Check sheet for the modelled part. Datum: model origin and axes. Units: mm. Round coordinates to 2 decimals unless told otherwise and drop trailing zeros. Loops run counter-clockwise (first coordinate to the right, second up) from the corner with the lowest first, then second, coordinate; pieces in that order, holes last. Notation, with made-up numbers: (77.25, -16) - (83.25, -16) arc R17 ccw to (83.25, -9) - close; hole circle Ø6 at (70.5, 10). An arc over 180 degrees is marked (long way). Return JSON: item names as keys, results as strings.
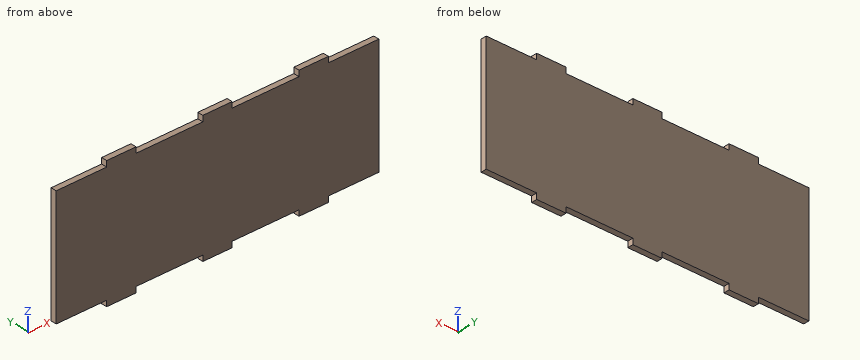
Autodesk Fusion 360 part; units mm, degrees
sketch "Skizze1" plane through (0, 0, 0) normal (0, 1, 0) x (1, 0, 0)
  line L0 (0, 0) -> (101, 0)
  line L1 (101, 0) -> (101, 40.6)
  line L2 (101, 40.6) -> (0, 40.6)
  line L3 (0, 40.6) -> (0, 0)
  line L4 (0, 0) -> (15.8, 0)
  line L5 (15.8, 0) -> (15.8, 1.8)
  line L6 (15.8, 1.8) -> (0, 1.8)
  line L7 (0, 1.8) -> (0, 0)
  line L8 (25, 0) -> (45.9, 0)
  line L9 (45.9, 0) -> (45.9, 1.8)
  line L10 (45.9, 1.8) -> (25, 1.8)
  line L11 (25, 1.8) -> (25, 0)
  line L12 (55.1, 0) -> (76, 0)
  line L13 (76, 0) -> (76, 1.8)
  line L14 (76, 1.8) -> (55.1, 1.8)
  line L15 (55.1, 1.8) -> (55.1, 0)
  line L16 (85.2, 0) -> (101, 0)
  line L17 (101, 0) -> (101, 1.8)
  line L18 (101, 1.8) -> (85.2, 1.8)
  line L19 (85.2, 1.8) -> (85.2, 0)
  line L20 (0, 40.6) -> (15.8, 40.6)
  line L21 (15.8, 40.6) -> (15.8, 38.8)
  line L22 (15.8, 38.8) -> (0, 38.8)
  line L23 (0, 38.8) -> (0, 40.6)
  line L24 (25, 40.6) -> (45.9, 40.6)
  line L25 (45.9, 40.6) -> (45.9, 38.8)
  line L26 (45.9, 38.8) -> (25, 38.8)
  line L27 (25, 38.8) -> (25, 40.6)
  line L28 (55.1, 40.6) -> (76, 40.6)
  line L29 (76, 40.6) -> (76, 38.8)
  line L30 (76, 38.8) -> (55.1, 38.8)
  line L31 (55.1, 38.8) -> (55.1, 40.6)
  line L32 (101, 40.6) -> (85.2, 40.6)
  line L33 (85.2, 40.6) -> (85.2, 38.8)
  line L34 (85.2, 38.8) -> (101, 38.8)
  line L35 (101, 38.8) -> (101, 40.6)
  dimension "d1" = 101
  dimension "d2" = 40.6
  dimension "d3" = 15.8
  dimension "d4" = 1.8
  dimension "d6" = 1.8
  dimension "d7" = 9.2
  dimension "d8" = 45.9
  dimension "d9" = 1.8
  dimension "d10" = 9.2
  dimension "d14" = 15.8
  dimension "d15" = 9.2
  dimension "d16" = 15.8
  dimension "d17" = 1.8
  dimension "d18" = 1.8
  dimension "d19" = 9.2
  dimension "d20" = 45.9
  dimension "d22" = 15.8
  dimension "d23" = 1.8
  dimension "d24" = 9.2
  dimension "d25" = 9.2
extrude "Extrusion1" add sketch "Skizze1" along normal blind 1.8 contours L0 L1 L2 L3 L5 L6 L9 L10 L11 L13 L14 L15 L18 L19 L21 L22 L25 L26 L27 L29 L30 L31 L33 L34
Q1. Depth check by flat-ended pin: P1, Ø0.5, axis at x = 31.5, y = 0.5, coming from the -Z side; P2, Ø0.5, axis at y = 1, z = -0.5, coming from the -X side; P3, Ø0.5, axis at x = 11, y = 1, coming from the +Z side. Enter the tip coordinate at first touch or a pass-through.
Answer key:
{"P1": "stops at z = -38.8", "P2": "stops at x = 15.8", "P3": "stops at z = -1.8"}
Q2. Scan line: probe 1 along Z at (x, y) = (32.5, 0.1). Record every from-to range of solid material in increasing order. Write a range as [from, to].
Answer key:
{"probe 1": "z = [-38.8, -1.8]"}
Q3. Sectioned sample at A-A (y = 1.5). Enter the section's corners in (x, z).
Answer key:
{"outline": "(0, -38.8) - (15.8, -38.8) - (15.8, -40.6) - (25, -40.6) - (25, -38.8) - (45.9, -38.8) - (45.9, -40.6) - (55.1, -40.6) - (55.1, -38.8) - (76, -38.8) - (76, -40.6) - (85.2, -40.6) - (85.2, -38.8) - (101, -38.8) - (101, -1.8) - (85.2, -1.8) - (85.2, 0) - (76, 0) - (76, -1.8) - (55.1, -1.8) - (55.1, 0) - (45.9, 0) - (45.9, -1.8) - (25, -1.8) - (25, 0) - (15.8, 0) - (15.8, -1.8) - (0, -1.8) - close"}
Q4. Sectioned sample at B-B (x = 93). Enter the section's corners in (y, z), plus the area to 3 significant figures.
Answer key:
{"outline": "(0, -38.8) - (1.8, -38.8) - (1.8, -1.8) - (0, -1.8) - close", "area": "66.6 mm²"}
